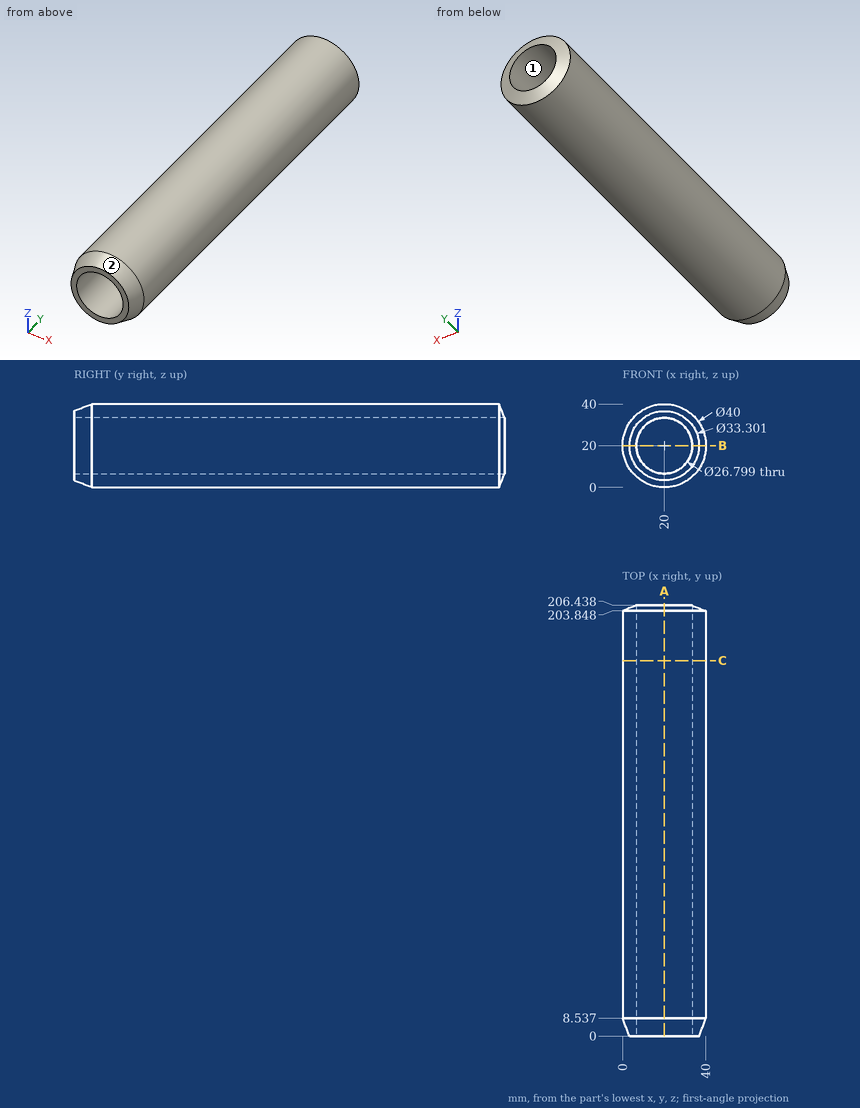
Job drawing, mm, ordinate dimensions from the low corner. One solid piece. Round coordinates to 2 decimals unless told otherwise and drop trailing zeros. Loops run counter-clockwise (first coordinate to the right, second up) from the corner with the lowest first, then second, coordinate; pieces in that order, holes last.
Item 1: Drop flat-ended pins along their axis: P1, Ø2, axis at x = 36, z = 30, coming from the +Y side (1 decimal); P2, Ø2, axis at x = 8, y = 94, coming from the +Z side; P3, Ø1.5, axis at x = 28.5, y = 172, coming from the -Z side. Give the stop position or say it passes through.
Item 2: Cut at A-A, the plane x = 20. Give the cut face in (y, z).
Item 3: Mould opens along Z. For the marked faces 1 and 2 say: +Z half, -Z half, draft (parallel to the pull), parting line (faces both ways), or undercut.
Item 4: Cut at B-B, the plane z = 20. Give the cut face in (x, y), then the cut area to 3 significant figures.
Item 5: Drill centre lines: line 1 (Z direction, x = 20, y = 65.5); line 2 (X direction, y = 122, z = 20.5); line 3 (X direction, y = 143, z = 27) (1 decimal). Where is each one in solid material? Low to high.
Item 6: Cut at C-C, the plane y = 180. Give the cut face in (x, z).
A:
1. P1: stops at y = 204.7
1. P2: stops at z = 36.7
1. P3: stops at z = 1.56
2. outline: (0, 3.35) - (8.54, 0) - (203.85, 0) - (206.44, 6.6) - (0, 6.6) - close; (0, 33.4) - (206.44, 33.4) - (203.85, 40) - (8.54, 40) - (0, 36.65) - close
3. face 1: undercut
3. face 2: parting line
4. outline: (0, 8.54) - (3.35, 0) - (6.6, 0) - (6.6, 206.44) - (0, 203.85) - close; (33.4, 0) - (36.65, 0) - (40, 8.54) - (40, 203.85) - (33.4, 206.44) - close
4. area: 2,680 mm2
5. line 1: z = 0 to 6.6, 33.4 to 40
5. line 2: x = 0.01 to 6.61, 33.39 to 39.99
5. line 3: x = 1.3 to 8.6, 31.4 to 38.7
6. outline: circle Ø40 at (20, 20); hole circle Ø26.8 at (20, 20)
